Check sheet for the modelled part. Datum: model origin and axes. Units: mm. Round coordinates to 2 decimals unless told otherwise and drop trailing zeros. Write each loop counter-clockwise with the first axis right and the second up, starting at its lowest first coordinate (ties: lowest second). Pieces come first, ordered by that corner, then holes. Notation, with made-up numbers: (-21, 43.5) -> (-12, 43.5) arc R8 cw to (-12, 47.5) -> close; hole circle Ø9 at (71, 57.5). An arc over 180 degrees is marked (long way). Answer as a JSON object with one key per item and string values. Group by question number.
Autodesk Inventor part; units mm, degrees
ref_plane "作業平面1" through (0, 0, 0) normal (0, 1, 0) x (-1, 0, 0)
ref_plane "YZ Plane" through (0, 0, 0) normal (1, 0, 0) x (0, 1, 0)
ref_plane "XY Plane" through (0, 0, 0) normal (0, 0, 1) x (1, 0, 0)
sketch "スケッチ1" plane through (0, 0, 0) normal (0, 0, 1) x (1, 0, 0)
  circle A0 centre (0, 0) radius 13.6
  dimension "d0" = 27.2
extrude "押し出し1" add sketch "スケッチ1" against normal blind 172.8
sketch "スケッチ3" plane through (0, 0, 0) normal (0, 0, 1) x (1, 0, 0)
  circle A0 centre (0, 0) radius 13.6
hole "穴1" at (0, 0, 0) direction (0, 0, -1) diameter 22.6 end through all
ref_plane "作業平面1" through (0, 0, 0) normal (0, 1, 0) x (-1, 0, 0)
sketch "スケッチ4" plane through (0, 0, 0) normal (0, 1, 0) x (-1, 0, 0)
  line L0 (-13.6, 0) -> (13.6, 0)
  arc A0 (-13.6, 0) -> (13.6, 0) centre (0, 0) ccw
  line L1 (13.6, 0) -> (-13.6, 0)
extrude "押し出し3" cut sketch "スケッチ4" along normal mid plane 27.2
sketch "スケッチ5" plane through (0, 0, 0) normal (0, 1, 0) x (-1, 0, 0)
  line L0 (-13.6, -172.8) -> (13.6, -172.8)
  arc A0 (13.6, -172.8) -> (-13.6, -172.8) centre (0, -172.8) ccw
  line L1 (-13.6, -172.8) -> (13.6, -172.8)
  point P0 (0, 0)
extrude "押し出し4" cut sketch "スケッチ5" along normal mid plane 27.2
properties part number "縦のパイプ"
(1) Go/stop test with flat-tipped pins: pin 1 Ø2 at (x, z) = (10, -115) entering from +Y; pin 2 Ø4 at (x, y) = (-1, 8) entering from -Z; pin 3 Ø8 at (x, y) = (-6, -10.5) entering from +Z; pin 4 Ø10 at (x, y) = (9, 6) entering from +Z. Record where each tip stops, or that it passes through.
(2) Section check A-A on x = 0. Record the cut outline in (y, z).
(3) Section check B-B on y = 0. Record the cut outline in (x, z), then the cut area to 3 significant figures.
(4) Release check for a two-part mould opening along Y. For faces 1 (the cylindrical face through (-11, -8, -85)), 2 (the cylindrical face through (-3.39, -10.78, -87.5)) record: pulls with the +Y half, pulls with the -Y half, needs draft (parallel to the pull), parting line crosses it, or undercut.
(5) Scan lines: line 1 along X through (y, z) = (0, -39); line 2 along Z through (x, y) = (-0.5, -12). Record each from-to range of solid material in increasing order.
(6) Section check C-C on z = -142.5. Record the cut outline in (x, y), then the cut area to 3 significant figures.
Data:
{
 "1": {"pin 1": "stops at y = 10.2", "pin 2": "passes through", "pin 3": "stops at z = -9.39", "pin 4": "stops at z = -3.28"},
 "2": {"outline": "(-13.6, -159.2) -> (-11.3, -159.2) -> (-11.3, -13.6) -> (-13.6, -13.6) -> close; (11.3, -159.2) -> (13.6, -159.2) -> (13.6, -13.6) -> (11.3, -13.6) -> close"},
 "3": {"outline": "(-13.6, -172.8) arc R13.6 cw to (-11.3, -165.23) -> (-11.3, -7.57) arc R13.6 cw to (-13.6, 0) -> close; (11.3, -165.23) arc R13.6 cw to (13.6, -172.8) -> (13.6, 0) arc R13.6 cw to (11.3, -7.57) -> close", "area": "748 mm²"},
 "4": {"face 1": "parting line crosses it", "face 2": "undercut"},
 "5": {"line 1": "x = -13.6 to -11.3, 11.3 to 13.6", "line 2": "z = -159.21 to -13.59"},
 "6": {"outline": "circle Ø27.2 at (0, 0); hole circle Ø22.6 at (0, 0)", "area": "180 mm²"}
}
